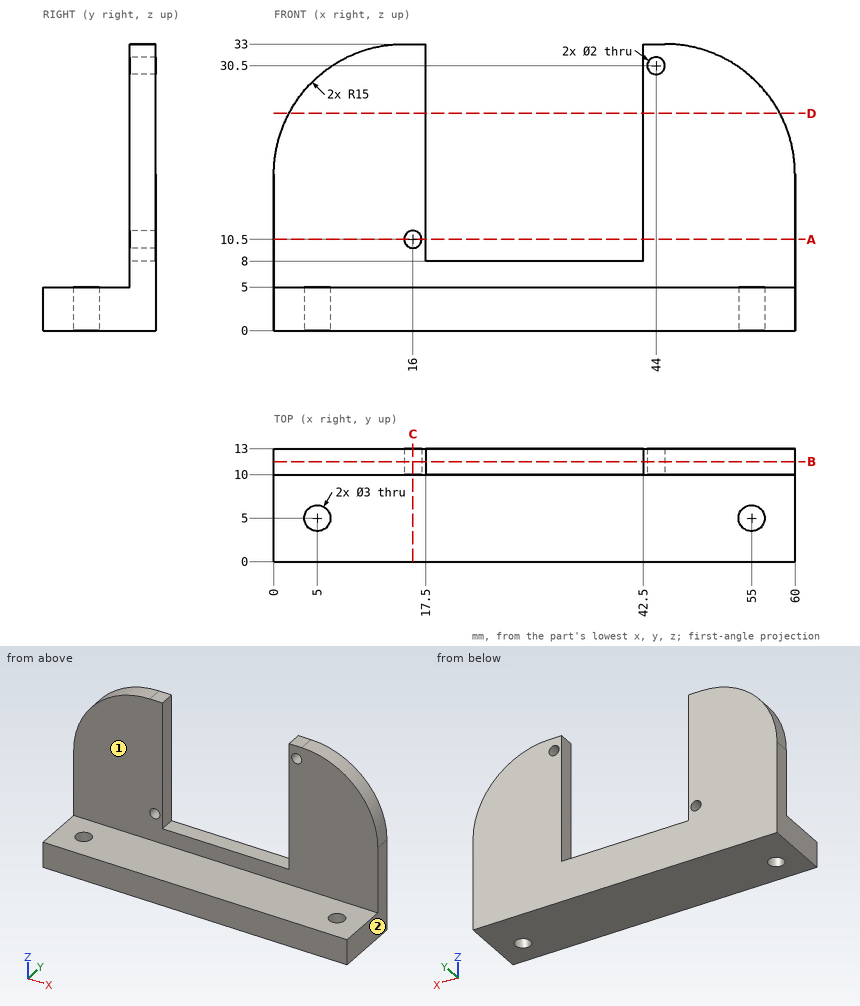
Input: dimensioned drawing with shaded views. Units: mm. Origin: part minimum x, y, z. A direction names the side the tool comes from. Coordinates: 2 decimals unless noted, no trailing zeros. Loops run counter-clockwise (first coordinate to the right, second up) from the corner with the lowest first, then second, coordinate; pieces in that order, holes last. Notation, with made-up numbers: M 72,-31.5 L 100,-31.5 A19 cw 100,-25.5 Z; hole C 29.25,-4 d1. An arc over 180 degrees is marked long. One line per item, written item: value. Start each with the question number.
1) Pin query (flat end, axial travel): P1, Ø1.5, axis at y = 12, z = 24.5, coming from the -X side; P2, Ø2.5, axis at y = 11.5, z = 24, coming from the +X side; P3, Ø3, axis at x = 44.5, y = 5, coming from the +Z side; P4, Ø1, axis at x = 52, y = 4.5, coming from the -Z side. Return the tip coordinate at first contact, or that it passes through.
2) Reachability of the marked faces 1 and 2 from +Z, -Z, +X, -X, +Y, -Y: full face, straight path, thin tool, end or side. Return the list, or none.
3) Material intervals for L1, parallel to Z at x = 44, y = 10.6; L2, parallel to Z at x = 16, y = 12.45; L3, parallel to Z at x = 25, y = 9.25, sorted ascending. Write a range as from..to.
4) Cut plane C-C (x = 16). Return loops of the section in (y, z).
5) Cut plane A-A (z = 10.5). Return loops of the section in (x, y).
6) Cut plane D-D (z = 25). Return loops of the section in (x, y), then the cut area to 3 significant figures.
7) Cut plane B-B (y = 11.5). Return loops of the section in (x, z), then the cut area to 3 significant figures.
Evaluation:
1. P1: x = 1.15
1. P2: x = 59.23
1. P3: z = 5
1. P4: z = 0
2. face 1: +Z, +X, -X, -Y
2. face 2: +Z, -Z, +X, +Y, -Y
3. L1: 0..29.5, 31.5..33
3. L2: 0..9.5, 11.5..33
3. L3: 0..5
4. outline: M 0,0 L 13,0 L 13,9.5 L 10,9.5 L 10,5 L 0,5 Z; M 10,11.5 L 13,11.5 L 13,33 L 10,33 Z
5. outline: M 0,10 L 15,10 L 15,13 L 0,13 Z; M 17,10 L 17.5,10 L 17.5,13 L 17,13 Z; M 42.5,10 L 60,10 L 60,13 L 42.5,13 Z
6. outline: M 1.73,10 L 17.5,10 L 17.5,13 L 1.73,13 Z; M 42.5,10 L 58.27,10 L 58.27,13 L 42.5,13 Z
6. area: 94.6 mm^2
7. outline: M 0,0 L 60,0 L 60,18 A15 ccw 45,33 L 42.5,33 L 42.5,8 L 17.5,8 L 17.5,33 L 15,33 A15 ccw 0,18 Z; hole C 16,10.5 d2; hole C 44,30.5 d2
7. area: 1,250 mm^2
